Input: dimensioned drawing with shaded views. Units: mm. Origin: part minimum x, y, z. Give positions to 0.01 mm unless a question says otherwise; leave off trailing zeros. Order: outer loops, then holes, each group sorted by start corner. A loop starts at its lowest first (then second) coordinate and runs counter-clockwise, first axis right, second up.
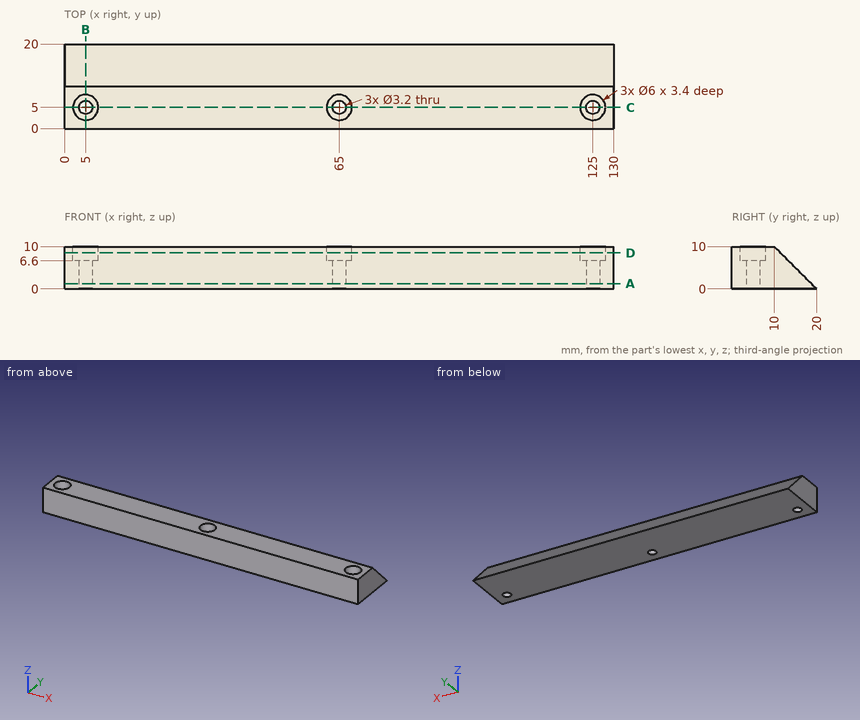
1) Cut plane A-A (z = 1.25). Return the cut outline in (x, y), then the cut area to 3 significant figures.
2) Cut plane C-C (y = 5). Return the cut outline in (x, z).
3) Line query: probe 1 along Y at (x, z) = (65, 5); probe 2 along Y at (x, z) = (65, 4.5); probe 3 along Z at (x, y) = (58.5, 14.5). Output: solid intervals per line, ascending.
4) Cut plane B-B (x = 5). Return the cut outline in (y, z), then the cut area to 3 significant figures.
5) Cut plane D-D (z = 8.5). Return the cut outline in (x, y), then the cut area to 3 significant figures.
6) First-contact query: P1, Ø3.5, axis at x = 5, y = 5, coming from the +Z side. Flat tip, straight axial feed; report the tip coordinate or a pass-through.
Geometry says:
1. outline: (0, 0) - (130, 0) - (130, 18.75) - (0, 18.75) - close; hole circle Ø3.2 at (5, 5); hole circle Ø3.2 at (65, 5); hole circle Ø3.2 at (125, 5)
1. area: 2,410 mm2
2. outline: (0, 0) - (3.4, 0) - (3.4, 6.6) - (2, 6.6) - (2, 10) - (0, 10) - close; (6.6, 0) - (63.4, 0) - (63.4, 6.6) - (62, 6.6) - (62, 10) - (8, 10) - (8, 6.6) - (6.6, 6.6) - close; (66.6, 0) - (123.4, 0) - (123.4, 6.6) - (122, 6.6) - (122, 10) - (68, 10) - (68, 6.6) - (66.6, 6.6) - close; (126.6, 0) - (130, 0) - (130, 10) - (128, 10) - (128, 6.6) - (126.6, 6.6) - close
3. probe 1: y = 0 to 3.4, 6.6 to 15
3. probe 2: y = 0 to 3.4, 6.6 to 15.5
3. probe 3: z = 0 to 5.5
4. outline: (0, 0) - (3.4, 0) - (3.4, 6.6) - (2, 6.6) - (2, 10) - (0, 10) - close; (6.6, 0) - (20, 0) - (10, 10) - (8, 10) - (8, 6.6) - (6.6, 6.6) - close
4. area: 108 mm2
5. outline: (0, 0) - (130, 0) - (130, 11.5) - (0, 11.5) - close; hole circle Ø6 at (5, 5); hole circle Ø6 at (65, 5); hole circle Ø6 at (125, 5)
5. area: 1,410 mm2
6. P1: stops at z = 6.6
